The listing builds one solid part. Answer for the finished solid, in the listing's coordinates (mm). A direction names the side the tool comes from. Coordinates: 2 decimals unless noted, no trailing zeros. Loops run counter-clockwise (first coordinate to the right, second up) from the corner with the lowest first, then second, coordinate; pieces in that order, holes last. Notation, with made-up numbers: M 66.25,69 L 76.25,69 A20 cw 76.25,78 Z; hole C 44.25,-12 d3. An arc over 180 degrees is marked long. Answer as a JSON object with one key per item and string values. Group by question number.
1. Straight lines are drawn through the part: L1, parallel to Y at x = 0, z = 1; L2, parallel to X at y = 3.25, z = 0.5. For each, find the intervals that lie inside material, in ascending order.
2. A cutting plane is placed at D-D on z = 10. Give the vertices of the cut face in (x, y).
3. Given pin 1 (12 mm diameter, centred on x = -9.5, z = -2, fed in from +Y); pin 2 (12.5 mm diameter, centred on x = 0, y = 0, fed in from -Z); pin 3 (12 mm diameter, centred on x = -0.5, z = 8.5, fed in from -Y); pin 4 (1.5 mm diameter, centred on y = 0.5, z = -6, fed in from +X), each flat-ended and moving along its own axis, determine where each tip first touches the part or whether it passes through.
4. For faces 1 (the face through (-1.172, -8.923, 6.591)), 2 (the face through (0.1, -10.2, -4)), determine the directions among +Z, -Z, +X, -X, +Y, -Y from which every point of the face is accessible in a straight line to the end or side of a thin tool.
5. A cutting plane is placed at C-C on z = -0.5. Give the vertices of the cut face in (x, y), and give its area (3 significant figures).
6. Determine the mould class of faces 3 (the face through (11.923, -3.755, -1.972)), 4 (the face through (6.466, 2.681, 2.832)), 5 (the face through (-2, -7, -9)) for opening direction X: released by +X, released by -X, zero draft, split by the parting line, or undercut.
from build123d import *

# Parameters (mm, degrees)
F0_W   = 2
F0_H   = 15
F0_W_2 = 3
F0_H_2 = 5
F2_R   = 1.99999


# Not quite as in the source:
# - a fillet or chamfer is up to 0.001 mm smaller than in the source, because OpenCascade refuses the exact size


with BuildPart() as f1:
    # F0 (on Front) → F1 (revolve)
    with BuildSketch(Plane.XZ):
        with Locations((8, 7.5)):
            Rectangle(F0_W, F0_H)
        Polygon((9, 0), (7, 0), (7, -4), (10, -4), (12.5, -4), (12.5, 0), align=None)
        with Locations((8.5, -6.5)):
            Rectangle(F0_W_2, F0_H_2)
    revolve(axis=Axis((0, 0, 7.5), (0, 0, -1)))

    # F2 (radius 2 in the source; OpenCascade refuses exactly that, so slightly less here)
    f2_edges = [f1.edges().sort_by_distance(p)[0] for p in [
        (-9, 0, 15),
    ]]
    fillet(f2_edges, radius=F2_R)


solid = f1.part
From the geometry:
{
 "1": {"L1": "y = -9 to -7, 7 to 9", "L2": "x = -8.39 to -6.2, 6.2 to 8.39"},
 "2": {"outline": "C 0,0 d18; hole C 0,0 d14"},
 "3": {"pin 1": "stops at y = 12", "pin 2": "passes through", "pin 3": "stops at y = -9", "pin 4": "stops at x = 10"},
 "4": {"face 1": "+Z", "face 2": "-Z"},
 "5": {"outline": "C 0,0 d25; hole C 0,0 d14", "area": "337 mm²"},
 "6": {"face 3": "split by the parting line", "face 4": "undercut", "face 5": "zero draft"}
}
